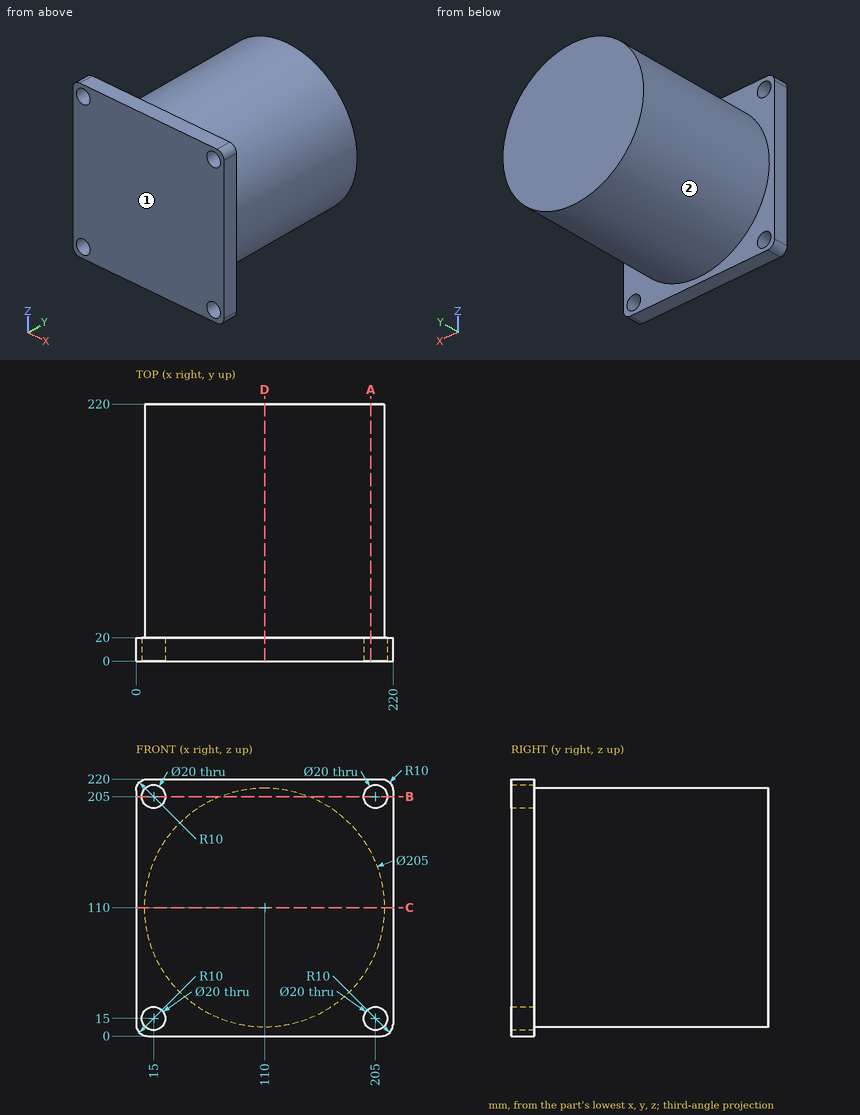
The drawing under review shows one solid part. Ordinate dimensions are in mm from its lowest x, y, z. A direction names the side the tool comes from. Round coordinates to 2 decimals unless told otherwise and drop trailing zeros. Order: outer loops, then holes, each group sorted by start corner. A loop starts at its lowest first (then second) coordinate and runs counter-clockwise, first axis right, second up. Notation, with made-up numbers: (-24, 78) -> (16, 78) arc R25 ccw to (16, 114) -> close; hole circle Ø10 at (33.5, 77). An arc over 180 degrees is marked (long way). Return JSON: item names as keys, results as strings.
1. Insertion check: P1, Ø1.5, axis at x = 40, y = 126.5, coming from the -Z side; P2, Ø5, axis at x = 115.5, y = 31, coming from the -Z side; P3, Ø1.5, axis at y = 99.5, z = 91.5, coming from the +X side. Each pin has a flat end and moves straight along its axis. Give the tip position at first contact, or say it passes through.
Answer block:
{"P1": "stops at z = 34.43", "P2": "stops at z = 7.54", "P3": "stops at x = 210.95"}
2. Take a section at A-A (x = 201). Write out the cut boundary in (y, z).
Answer block:
{"outline": "(0, 0) -> (20, 0) -> (20, 5.83) -> (0, 5.83) -> close; (0, 24.17) -> (20, 24.17) -> (20, 62.83) -> (220, 62.83) -> (220, 157.17) -> (20, 157.17) -> (20, 195.83) -> (0, 195.83) -> close; (0, 214.17) -> (20, 214.17) -> (20, 220) -> (0, 220) -> close"}
3. Take a section at C-C (z = 110). Write out the cut boundary in (x, y).
Answer block:
{"outline": "(0, 0) -> (220, 0) -> (220, 20) -> (212.5, 20) -> (212.5, 220) -> (7.5, 220) -> (7.5, 20) -> (0, 20) -> close"}
4. Take a section at B-B (z = 205). Write out the cut boundary in (x, y).
Answer block:
{"outline": "(0, 0) -> (5, 0) -> (5, 20) -> (0, 20) -> close; (25, 0) -> (195, 0) -> (195, 20) -> (148.49, 20) -> (148.49, 220) -> (71.51, 220) -> (71.51, 20) -> (25, 20) -> close; (215, 0) -> (220, 0) -> (220, 20) -> (215, 20) -> close"}
5. For the marked faces 1 and 2, list the 3-axis set-ups (+Z, -Z, +X, -X, +Y, -Y) from which the entire face can be reached by the end or side of a thin tool; tool diameter is ignored.
Answer block:
{"face 1": "+Z, -Z, +X, -X, -Y", "face 2": "+Y"}
6. For L1, parallel to X at y = 7.5, z = 205; L2, parallel to Y at x = 208, z = 58; L3, parallel to Z at x = 166, y = 62, list the stretches that pass through material, from the lowest coordinate up. Write a range as [from, to].
Answer block:
{"L1": "x = [0, 5], [25, 195], [215, 220]", "L2": "y = [0, 20]", "L3": "z = [24.15, 195.85]"}
7. Take a section at D-D (x = 110). Write out the cut boundary in (y, z), then the cut area to 3 significant figures.
Answer block:
{"outline": "(0, 0) -> (20, 0) -> (20, 7.5) -> (220, 7.5) -> (220, 212.5) -> (20, 212.5) -> (20, 220) -> (0, 220) -> close", "area": "45,400 mm²"}
